The model under review builds one solid part; all positions refer to its coordinate system, in mm. A direction names the side the tool comes from. Round coordinates to 2 decimals unless told otherwise and drop trailing zeros. Order: outer loops, then holes, each group sorted by start corner. A loop starts at its lowest first (then second) coordinate and runs counter-clockwise, first axis right, second up. Notation, with made-up numbers: M 84.5,-21.75 L 136.5,-21.75 A24 ccw 136.5,15.25 Z; hole C 4,4.5 d1. An arc over 180 degrees is marked long. Answer as a JSON object with one key per item and string values. Group by question number.
1) To check wall thickness, follow line 1 (X direction, y = 7, z = 6.5); line 2 (Y direction, x = 0.6, z = 30.48). State the ranges of each line that lie inside material, in increasing order.
2) Consider section A-A, the plane y = 0. Write out the cut boundary in (x, z) (3 decimals), then the cut area to 3 significant figures.
3) The part is to be moulded in two halves that separate along Y. For faces 1 (the flat face through (1, -11.112, 9)), 2 (the cylindrical face through (0.644, -1.468, 32.395)), 3 (the cylindrical face through (0.573, -0.156, 0.543)), say which applies: +Y half, -Y half, draft (parallel to the pull), parting line (faces both ways), or undercut.
4) Consider section D-D, the plane y = 8.25. Write out the cut boundary in (x, z) (3 decimals).
5) Insertion check: pin 1 Ø6 at (x, y) = (11, -4) entering from +Z; pin 2 Ø6.5 at (y, z) = (0, 30.48) entering from -X; pin 3 Ø3 at (x, y) = (30.48, 0) entering from -Z; pin 4 Ø8 at (y, z) = (-6, 15.5) entering from +X. Each pin has a flat end and moves straight along its axis. Give the tip position at first contact, or say it passes through.
6) For faces 4 (the flat face through (1.27, 0, 20)), 5 (the flat face through (0, 0, 20)), list the 3-axis set-ups (+Z, -Z, +X, -X, +Y, -Y) from which the entire face can be reached by the end or side of a thin tool; tool diameter is ignored.
7) Consider section B-B, the plane x = 30.48. Write out the cut boundary in (y, z).
8) Consider section C-C, the plane z = 30.48. Write out the cut boundary in (x, y), then the cut area to 3 significant figures.
```python
from build123d import *

# Parameters (mm, degrees)
EXTRUDE_THIN1_START     = -11.1125
EXTRUDE_THIN1_DEPTH     = 22.225
SKETCH4_R               = 2.413
EXTRUDE3_DEPTH          = 55.143758239
SKETCH6_R               = 2.413
CUT_EXTRUDE1_DEPTH      = 56.015521957
CUT_EXTRUDE2_DEPTH      = 55.143758239
CUT_EXTRUDE2_DEPTH_BACK = 55.143758239
CUT_EXTRUDE3_DEPTH      = 56.015521957
CUT_EXTRUDE3_DEPTH_BACK = 56.015521957


# Read off the part's stored shape, not the designer's step: Extrude-Thin1
with BuildPart() as part:
    # Extrude-Thin1 outline → Extrude-Thin1 (new body)
    with BuildSketch(Plane(origin=(0, 0, 0), x_dir=(1, 0, 0), z_dir=(0, 1, 0)).offset(EXTRUDE_THIN1_START)):
        with BuildLine():
            Line((1.905, -1.27), (38.1, -1.27))
            Line((38.1, -1.27), (38.1, 0))
            Line((38.1, 0), (1.905, 0))
            ThreePointArc((1.905, 0), (0.557961582, -0.557961582), (0, -1.905))
            Line((0, -1.905), (0, -38.1))
            Line((0, -38.1), (1.27, -38.1))
            Line((1.27, -38.1), (1.27, -1.905))
            ThreePointArc((1.27, -1.905), (1.455987194, -1.455987194), (1.905, -1.27))
        make_face()
    extrude(amount=EXTRUDE_THIN1_DEPTH)

    # Sketch4 → Extrude3 (cut, through all)
    with BuildSketch(Plane(origin=(1.27, 0, 0), x_dir=(0, 0, -1), z_dir=(1, 0, 0))):
        with Locations((-30.48, 0)):
            Circle(SKETCH4_R)
    extrude(amount=-EXTRUDE3_DEPTH, mode=Mode.SUBTRACT)

    # Sketch6 → Cut-Extrude1 (cut, through all)
    with BuildSketch(Plane.XY):
        with Locations(Location((30.48, 0, 0), (0, 0, 180))):
            Circle(SKETCH6_R)
    extrude(amount=CUT_EXTRUDE1_DEPTH, mode=Mode.SUBTRACT)

    # Sketch8 → Cut-Extrude2 (cut, two sides: drawn at the far end of the back side and taken through both)
    with BuildSketch(Plane(origin=(1.27, 0, 0), x_dir=(0, 0, -1), z_dir=(1, 0, 0)).offset(-CUT_EXTRUDE2_DEPTH_BACK)):
        with BuildLine():
            Line((38.510183264, 64.402949948), (-32.54375, 11.1125))
            ThreePointArc((-32.54375, 11.1125), (-38.1, 0), (-32.54375, -11.1125))
            Line((-32.54375, -11.1125), (38.510183264, -64.402949948))
            Line((38.510183264, -64.402949948), (-139.124649895, -64.402949948))
            Line((-139.124649895, -64.402949948), (-139.124649895, 64.402949948))
            Line((-139.124649895, 64.402949948), (38.510183264, 64.402949948))
        make_face()
    extrude(amount=CUT_EXTRUDE2_DEPTH + CUT_EXTRUDE2_DEPTH_BACK, mode=Mode.SUBTRACT)

    # Sketch9 → Cut-Extrude3 (cut, two sides: drawn at the far end of the back side and taken through both)
    with BuildSketch(Plane.XY.offset(-CUT_EXTRUDE3_DEPTH_BACK)):
        with BuildLine():
            Line((-38.510183264, 64.402949948), (32.54375, 11.1125))
            ThreePointArc((32.54375, 11.1125), (38.1, 0), (32.54375, -11.1125))
            Line((32.54375, -11.1125), (-38.510183264, -64.402949948))
            Line((-38.510183264, -64.402949948), (139.124649895, -64.402949948))
            Line((139.124649895, -64.402949948), (139.124649895, 64.402949948))
            Line((139.124649895, 64.402949948), (-38.510183264, 64.402949948))
        make_face()
    extrude(amount=CUT_EXTRUDE3_DEPTH + CUT_EXTRUDE3_DEPTH_BACK, mode=Mode.SUBTRACT)


solid = part.part
```
Results list:
{
 "1": {"line 1": "0 to 1.27", "line 2": "-11.11 to -2.41, 2.41 to 11.11"},
 "2": {"outline": "M 0,1.905 A1.905 ccw 1.905,0 L 28.067,0 L 28.067,1.27 L 1.905,1.27 A0.635 cw 1.27,1.905 L 1.27,28.067 L 0,28.067 Z; M 0,32.893 L 1.27,32.893 L 1.27,38.1 L 0,38.1 Z; M 32.893,0 L 38.1,0 L 38.1,1.27 L 32.893,1.27 Z", "area": "82.2 mm^2"},
 "3": {"face 1": "-Y half", "face 2": "undercut", "face 3": "draft"},
 "4": {"outline": "M 0,1.905 A1.905 ccw 1.905,0 L 35.385,0 L 35.385,1.27 L 1.905,1.27 A0.635 cw 1.27,1.905 L 1.27,35.385 L 0,35.385 Z"},
 "5": {"pin 1": "z = 1.27", "pin 2": "x = 0", "pin 3": "through", "pin 4": "x = 1.27"},
 "6": {"face 4": "+Z, +X, +Y, -Y", "face 5": "+Z, -Z, -X, +Y, -Y"},
 "7": {"outline": "M -11.11,0 L -2.41,0 L -2.41,1.27 L -11.11,1.27 Z; M 2.41,0 L 11.11,0 L 11.11,1.27 L 2.41,1.27 Z"},
 "8": {"outline": "M 0,-11.11 L 1.27,-11.11 L 1.27,-2.41 L 0,-2.41 Z; M 0,2.41 L 1.27,2.41 L 1.27,11.11 L 0,11.11 Z", "area": "22.1 mm^2"}
}
